For this review, use the dimensioned drawing (mm, ordinates from the lowest corner) and the shaded views. Give positions to 0.01 mm unless a question says otherwise; leave off trailing zeros. Write each loop counter-clockwise with the first axis right and the second up, starting at its lowest first coordinate (ties: lowest second). Pieces come first, ordered by that corner, then holes. Notation, with made-up numbers: M 26.25,88 L 50.25,88 A36 ccw 50.25,127 Z; hole C 58,69 d10. An arc over 180 degrees is marked long. Answer in a Markdown table with one row per item.
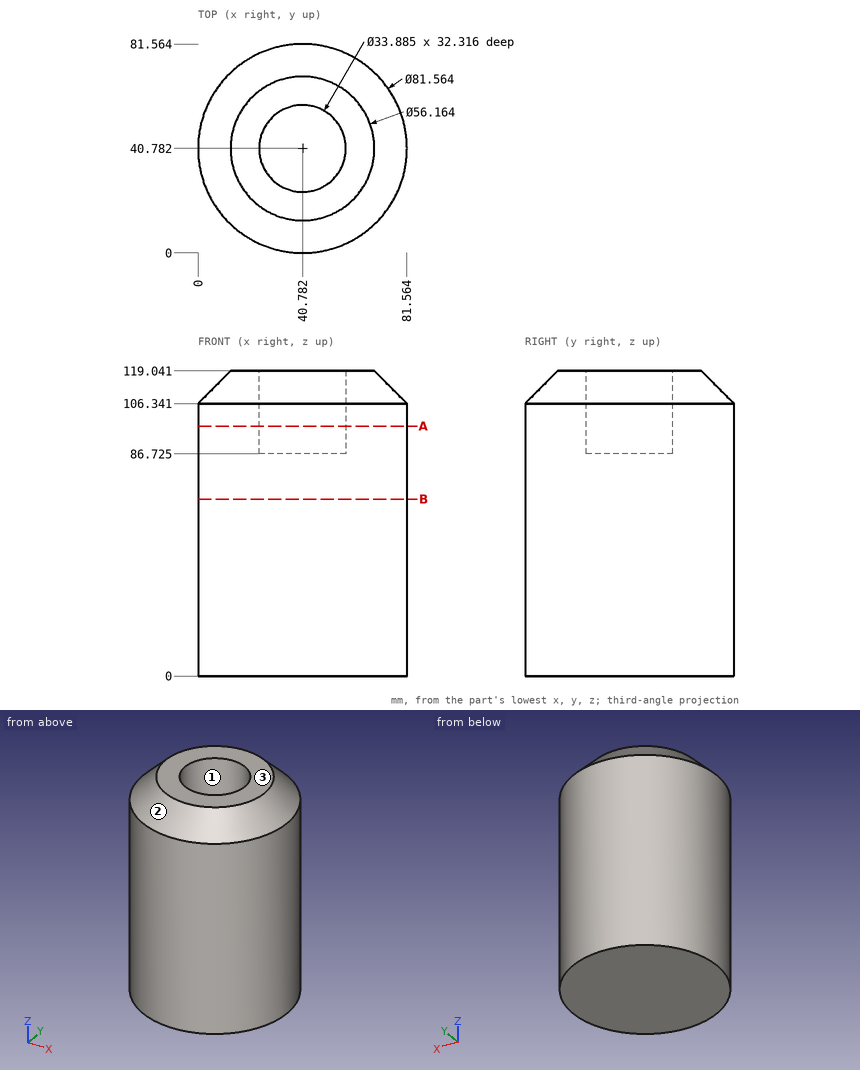
1) Insertion check: P1, Ø1, axis at y = 48.5, z = 52.5, coming from the -X side; P2, Ø12, axis at x = 23.5, z = 98.5, coming from the +Y side; P3, Ø1, axis at y = 53.5, z = 66.5, coming from the +X side. Each pin has a flat end and moves straight along its axis. Give the tip position at first contact, or say it passes through.
Geometry says:
| item | result |
|---|---|
| P1 | x = 0.64 |
| P2 | y = 79.97 |
| P3 | x = 79.69 |
2) Add section A-A (z = 97.5). Write out the cut boundary in (x, y) (1 decimal), and give its area (3 significant figures).
Geometry says:
| item | result |
|---|---|
| outline | C 40.8,40.8 d81.6; hole C 40.8,40.8 d33.9 |
| area | 4,320 mm^2 |
3) To check wall thickness, follow probe 1 along Y at (x, z) = (31, 77); probe 2 along X at (y, z) = (53, 20); probe 3 along X at (y, z) = (36, 55). State the ranges of each line that lie inside material, in increasing order. Write a range as [from, to].
Geometry says:
| item | result |
|---|---|
| probe 1 | [1.19, 80.37] |
| probe 2 | [1.87, 79.69] |
| probe 3 | [0.28, 81.28] |
4) Add section B-B (z = 69). Write out the cut boundary in (x, y).
Geometry says:
| item | result |
|---|---|
| outline | C 40.78,40.78 d81.56 |
5) The part is to be moulded in two halves that separate along Y. For the marked faces 1, 2 and 3, say which applies: released by +Y, released by -Y, zero draft, split by the parting line, or undercut.
Geometry says:
| item | result |
|---|---|
| face 1 | undercut |
| face 2 | split by the parting line |
| face 3 | zero draft |
